Source: three-view drawing plus pictorial views. Frame: mm from the lowest corner of the part. Coordinates: 2 decimals unless noted, no trailing zeros. Write each loop counter-clockwise with the first axis right and the second up, starting at its lowest first coordinate (ties: lowest second). Pieces come first, ordered by that corner, then holes. Notation, with made-up numbers: (16, 47) - (37, 47) arc R22 ccw to (37, 86) - close; hole circle Ø1 at (-25, 31). An arc over 180 degrees is marked (long way). One line per item, written item: value.
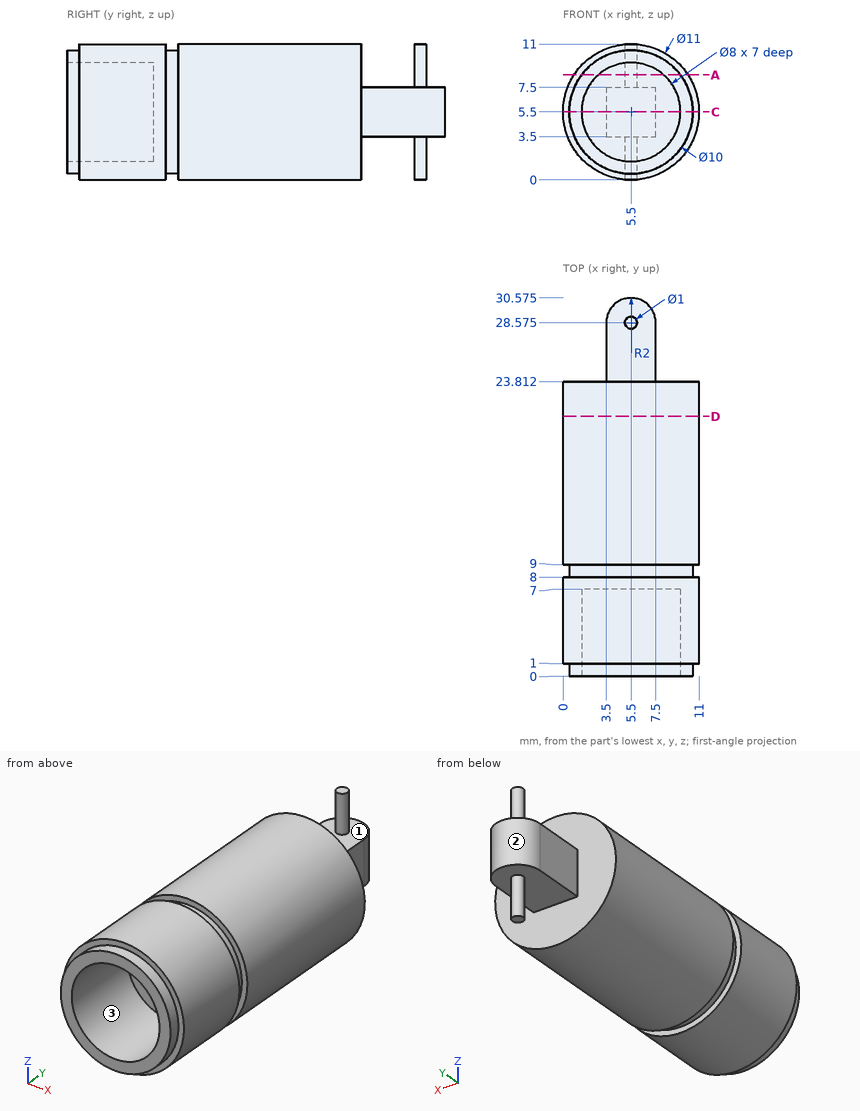
1) Material intervals for line 1 (X direction, y = 3.25, z = 5.5); line 2 (Y direction, x = 4, z = 8.25); line 3 (Y direction, x = 5.5, z = 7.75) (1 decimal), sorted ascending.
Values found:
line 1: 0 to 1.5, 9.5 to 11
line 2: 7 to 23.81
line 3: 7 to 23.8, 28.1 to 29.1
2) Section query A-A on z = 8.5. Output: boundary loops of the cut face in (x, y) (1 decimal).
Values found:
outline: (0.9, 1) - (1.5, 1) - (1.5, 0) - (2.9, 0) - (2.9, 7) - (8.1, 7) - (8.1, 0) - (9.5, 0) - (9.5, 1) - (10.1, 1) - (10.1, 8) - (9.5, 8) - (9.5, 9) - (10.1, 9) - (10.1, 23.8) - (0.9, 23.8) - (0.9, 9) - (1.5, 9) - (1.5, 8) - (0.9, 8) - close; circle Ø1 at (5.5, 28.6)
3) Contact query for flat-ended pins moving along their axis: P1, Ø2, axis at y = 20, z = 3.5, coming from the +X side; P2, Ø5.5, axis at x = 8, z = 3, coming from the +Y side (1 decimal); P3, Ø3.5, axis at x = 6, z = 3.5, coming from the -Y side; P4, Ø2, axis at y = 27, z = 5.5, coming from the -X side. Output: stop coordinate, or through.
Values found:
P1: x = 10.91
P2: y = 30.6
P3: y = 7
P4: x = 3.5
4) Draft query along Y for the marked faces 1, 2 and 3. Return one class per face: released by +Y, released by -Y, zero draft, split by the parting line, or undercut.
Values found:
face 1: undercut
face 2: released by +Y
face 3: zero draft
5) Section query C-C on z = 5.5. Output: boundary loops of the cut face in (x, y) (1 decimal), then the cut area to 3 significant figures.
Values found:
outline: (0, 1) - (0.5, 1) - (0.5, 0) - (1.5, 0) - (1.5, 7) - (9.5, 7) - (9.5, 0) - (10.5, 0) - (10.5, 1) - (11, 1) - (11, 8) - (10.5, 8) - (10.5, 9) - (11, 9) - (11, 23.8) - (7.5, 23.8) - (7.5, 28.6) arc R2 ccw to (3.5, 28.6) - (3.5, 23.8) - (0, 23.8) - (0, 9) - (0.5, 9) - (0.5, 8) - (0, 8) - close
area: 229 mm2
6) Section query D-D on y = 21. Output: boundary loops of the cut face in (x, z).
Values found:
outline: circle Ø11 at (5.5, 5.5)
